Answer from the drawing. Dimensions are ordinates in mm from the lowest x, y and z of the part. A direction names the side the tool comes from. Round coordinates to 2 decimals unless told otherwise and drop trailing zeros. Order: outer loops, then holes, each group sorted by start corner. A loop starts at its lowest first (then second) coordinate and runs counter-clockwise, first axis right, second up. Notation, with made-up numbers: (13.5, 29) -> (32.5, 29) arc R18 cw to (32.5, 36) -> close; hole circle Ø1 at (89.25, 63.5). An arc over 180 degrees is marked (long way). Use a Markdown table: item, result. Add a question column.
1. The mould has two halves that part along Z. Classify the marked faces 1, 2 and 3: +Z half, -Z half, draft (parallel to the pull), parting line (faces both ways), or undercut.
2. Consider L1, parallel to Y at x = 72, z = 4; L2, parallel to X at y = 18.5, z = 0.75; L3, parallel to Y at x = 40, z = 2.5. Determine where each line is inside the solid, lowest interval first. Write a range as [from, to].
3. Section D-D, the plane x = 64 is taken. Give the vertices of the cut face in (y, z), then the cut area to 3 significant figures.
4. Section B-B, the plane y = 21.5 is taken. Give the vertices of the cut face in (x, z).
5. For the marked faces 4, 5 and 6, determine the directions among +Z, -Z, +X, -X, +Y, -Y from which every point of the face is accessible in a straight line to the end or side of a thin tool.
6. Section C-C, the plane z = 4.75 is taken. Give the vertices of the cut face in (x, y), then the cut area to 3 significant figures.
7. Section A-A, the plane x = 8 is taken. Give the vertices of the cut face in (y, z).
8. Given pin 1 (2 mm diameter, centred on y = 6.5, z = 3.5, fed in from +X); pin 2 (3 mm diameter, centred on x = 4, z = 4.5, fed in from -Y), each flat-ended and moving along its own axis, determine where each tip first touches the part or whether it passes through.
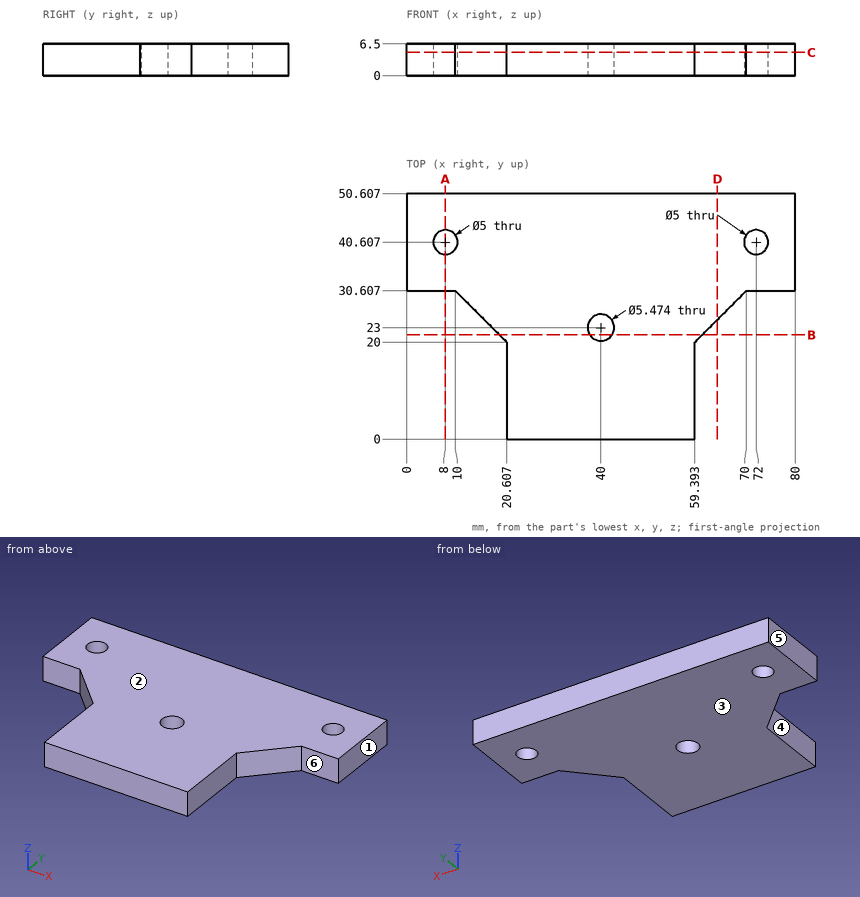
Verdict:
| question | item | result |
|---|---|---|
| 1 | face 1 | draft |
| 1 | face 2 | +Z half |
| 1 | face 3 | -Z half |
| 2 | L1 | y = [30.61, 38.11], [43.11, 50.61] |
| 2 | L2 | x = [20.61, 59.39] |
| 2 | L3 | y = [0, 20.26], [25.74, 50.61] |
| 3 | outline | (24.61, 0) -> (50.61, 0) -> (50.61, 6.5) -> (24.61, 6.5) -> close |
| 3 | area | 169 mm2 |
| 4 | outline | (19.11, 0) -> (37.71, 0) -> (37.71, 6.5) -> (19.11, 6.5) -> close; (42.29, 0) -> (60.89, 0) -> (60.89, 6.5) -> (42.29, 6.5) -> close |
| 5 | face 4 | +Z, -Z, -X, -Y |
| 5 | face 5 | +Z, -Z, -X, +Y, -Y |
| 5 | face 6 | +Z, -Z, +X, -Y |
| 6 | outline | (0, 30.61) -> (10, 30.61) -> (20.61, 20) -> (20.61, 0) -> (59.39, 0) -> (59.39, 20) -> (70, 30.61) -> (80, 30.61) -> (80, 50.61) -> (0, 50.61) -> close; hole circle Ø5 at (8, 40.61); hole circle Ø5.47 at (40, 23); hole circle Ø5 at (72, 40.61) |
| 6 | area | 2,840 mm2 |
| 7 | outline | (30.61, 0) -> (38.11, 0) -> (38.11, 6.5) -> (30.61, 6.5) -> close; (43.11, 0) -> (50.61, 0) -> (50.61, 6.5) -> (43.11, 6.5) -> close |
| 8 | pin 1 | stops at x = 59.39 |
| 8 | pin 2 | stops at y = 30.61 |
